Source: CAD feature listing. Evaluate the final solid. Frame: model axes, mm. A direction names the side the tool comes from. Give positions to 0.01 mm unless a question says otherwise; leave off trailing zeros. Order: outer loops, then holes, each group sorted by start corner. A loop starts at its lowest first (then second) coordinate and runs counter-clockwise, first axis right, second up. Notation, with made-up numbers: (-22.75, 62) -> (2.25, 62) arc R22 cw to (2.25, 84) -> close; hole circle Ø6 at (79, -27.5). An arc over 180 degrees is marked (long way). Use one line per item in the form item = value. Start each with the question number.
from build123d import *

# Parameters (mm, degrees)
SKETCH1_W           = 18.4
SKETCH1_H           = 15.9
BOSS_EXTRUDE1_DEPTH = 1.5
SKETCH2_W           = 2.5
SKETCH2_H           = 15.2
BOSS_EXTRUDE2_DEPTH = 2.6
BOSS_EXTRUDE3_START = -5.1
SKETCH3_W           = 0.64
SKETCH3_H           = 0.64
BOSS_EXTRUDE3_DEPTH = 11
SKETCH5_W           = 4.4
SKETCH5_H           = 5.1
SKETCH5_W_2         = 1.2
SKETCH5_H_2         = 2
BOSS_EXTRUDE4_DEPTH = 1.1
SKETCH6_W           = 1.2
SKETCH6_H           = 1.2
BOSS_EXTRUDE5_DEPTH = 1
SKETCH7_W           = 3.4
SKETCH7_H           = 1.8
BOSS_EXTRUDE6_DEPTH = 1.9
SKETCH8_W           = 1.2
SKETCH8_H           = 1.2
CUT_EXTRUDE1_DEPTH  = 0.05
SKETCH9_W           = 1.2
SKETCH9_H           = 1.05
CUT_EXTRUDE2_DEPTH  = 0.05
SKETCH10_W          = 1.2
SKETCH10_H          = 1.05
CUT_EXTRUDE3_DEPTH  = 0.05


with BuildPart() as part:
    # Sketch1 → Boss-Extrude1 (new body)
    with BuildSketch(Plane(origin=(0, 0, 0), x_dir=(1, 0, 0), z_dir=(0, 1, 0))):
        Rectangle(SKETCH1_W, SKETCH1_H)
    extrude(amount=-BOSS_EXTRUDE1_DEPTH)

    # Sketch2 → Boss-Extrude2 (add)
    with BuildSketch(Plane.XZ.offset(1.5)):
        with Locations((-7.6, 0)):
            Rectangle(SKETCH2_W, SKETCH2_H)
    boss_extrude2 = extrude(amount=BOSS_EXTRUDE2_DEPTH)

    # Sketch3 → Boss-Extrude3 (add)
    with BuildSketch(Plane(origin=(0, -4.1, 0), x_dir=(-1, 0, 0), z_dir=(0, -1, 0)).offset(BOSS_EXTRUDE3_START)):
        with Locations((7.6, -6.35)):
            Rectangle(SKETCH3_W, SKETCH3_H)
        with Locations((7.6, -3.81)):
            Rectangle(SKETCH3_W, SKETCH3_H)
        with Locations((7.6, -1.27)):
            Rectangle(SKETCH3_W, SKETCH3_H)
        with Locations((7.6, 1.27)):
            Rectangle(SKETCH3_W, SKETCH3_H)
        with Locations((7.6, 6.35)):
            Rectangle(SKETCH3_W, SKETCH3_H)
        with Locations((7.6, 3.81)):
            Rectangle(SKETCH3_W, SKETCH3_H)
    boss_extrude3 = extrude(amount=BOSS_EXTRUDE3_DEPTH)

    # Mirror1: Boss-Extrude2, Boss-Extrude3 across plane
    add(boss_extrude2.mirror(Plane(origin=(0, 0, 0), x_dir=(0, 0, 1), z_dir=(1, 0, 0))))
    add(boss_extrude3.mirror(Plane(origin=(0, 0, 0), x_dir=(0, 0, 1), z_dir=(1, 0, 0))))

    # Sketch5 → Boss-Extrude4 (add)
    with BuildSketch(Plane(origin=(0, 0, 0), x_dir=(1, 0, 0), z_dir=(0, 1, 0))):
        with Locations((-1.5, 0.5)):
            Rectangle(SKETCH5_W, SKETCH5_H)
        with Locations((4.5979, 0.1395)):
            Rectangle(SKETCH5_W_2, SKETCH5_H_2)
        with Locations((4.5979, 5.5766)):
            Rectangle(SKETCH5_W_2, SKETCH5_H_2)
    extrude(amount=BOSS_EXTRUDE4_DEPTH)

    # Sketch6 → Boss-Extrude5 (add)
    with BuildSketch(Plane(origin=(0, 0, 0), x_dir=(1, 0, 0), z_dir=(0, 1, 0))):
        with Locations((-0.3788, 6.0122)):
            Rectangle(SKETCH6_W, SKETCH6_H)
    extrude(amount=BOSS_EXTRUDE5_DEPTH)

    # Sketch7 → Boss-Extrude6 (add)
    with BuildSketch(Plane(origin=(0, 0, 0), x_dir=(1, 0, 0), z_dir=(0, 1, 0))):
        with Locations((-2.8238, -5.3484)):
            Rectangle(SKETCH7_W, SKETCH7_H)
    extrude(amount=BOSS_EXTRUDE6_DEPTH)

    # Sketch8 → Cut-Extrude1 (cut)
    with BuildSketch(Plane(origin=(0, 1.1, 0), x_dir=(1, 0, 0), z_dir=(0, 1, 0))):
        with Locations((4.5979, 5.5766)):
            Rectangle(SKETCH8_W, SKETCH8_H)
        with Locations((4.5979, 0.1395)):
            Rectangle(SKETCH8_W, SKETCH8_H)
    extrude(amount=-CUT_EXTRUDE1_DEPTH, mode=Mode.SUBTRACT)

    # Sketch9 → Cut-Extrude2 (cut)
    with BuildSketch(Plane.ZY.offset(-3.9979)):
        with Locations((-0.1395, 0.525)):
            Rectangle(SKETCH9_W, SKETCH9_H)
        with Locations((-5.5766, 0.525)):
            Rectangle(SKETCH9_W, SKETCH9_H)
    extrude(amount=-CUT_EXTRUDE2_DEPTH, mode=Mode.SUBTRACT)

    # Sketch10 → Cut-Extrude3 (cut)
    with BuildSketch(Plane(origin=(5.1979, 0, 0), x_dir=(0, 0, -1), z_dir=(1, 0, 0))):
        with Locations((0.1395, 0.525)):
            Rectangle(SKETCH10_W, SKETCH10_H)
        with Locations((5.5766, 0.525)):
            Rectangle(SKETCH10_W, SKETCH10_H)
    extrude(amount=-CUT_EXTRUDE3_DEPTH, mode=Mode.SUBTRACT)


solid = part.part
1) Cut plane B-B, the plane z = -2.25. Return the cut outline in (x, y), plus the area to 3 significant figures.
2) Reachability of faces 1 (the face through (4.6, 0.5, -4.577)), 2 (the face through (4.6, 0.5, -6.577)), 3 (the face through (0.7, 0.5, -0.5)), 4 (the face through (-2, 1.1, -1)), 5 (the face through (0, 1, -6)) from +Z, -Z, +X, -X, +Y, -Y: full face, straight path, thin tool, end or side. Return the list, or none.
3) Cut plane C-C, the plane x = -1.5. Return the cut outline in (y, z), plus the area to 3 significant figures.
4) Material intervals for probe 1 along X at (y, z) = (0.25, -6.5); probe 2 along X at (y, z) = (-1.75, 4); probe 3 along Y at (x, z) = (2, 7), sorted ascending.
5) Draft query along X for faces 6 (the face through (8.85, -3, 0)), 7 (the face through (6.35, -3, 0)), 8 (the face through (4.6, 1.05, -0.1)), 9 (the face through (-3.7, 0.5, -0.5)). Return one class per face: +X half, -X half, draft (parallel to the pull), parting line (faces both ways), or undercut.
6) Pin query (flat end, axial travel): pin 1 (1.5 mm diameter, centred on y = -2.5, z = 0.5, fed in from -X); pin 2 (4 mm diameter, centred on x = -1.5, z = 5.5, fed in from -Y); pin 3 (0.5 mm diameter, centred on y = 0.5, z = -6.5, fed in from +X). Return the tip coordinate at first contact, or that it passes through.
7) Cut plane A-A, the plane y = -3.75. Return the cut outline in (x, z).
8) Cut plane D-D, the plane x = 4.5. Return the cut outline in (y, z), plus the area to 3 significant figures.
Output values:
q1.outline = (-9.2, -1.5) -> (-8.85, -1.5) -> (-8.85, -4.1) -> (-6.35, -4.1) -> (-6.35, -1.5) -> (6.35, -1.5) -> (6.35, -4.1) -> (8.85, -4.1) -> (8.85, -1.5) -> (9.2, -1.5) -> (9.2, 0) -> (0.7, 0) -> (0.7, 1.1) -> (-3.7, 1.1) -> (-3.7, 0) -> (-9.2, 0) -> close
q1.area = 45.4 mm^2
q2.face_1 = +X, -X, +Y
q2.face_2 = -Z, +Y
q2.face_3 = +Z, -Z, +Y
q2.face_4 = -Z, +X, -X, +Y
q2.face_5 = -Z, -X, +Y
q3.outline = (-1.5, -7.95) -> (0, -7.95) -> (0, -3.05) -> (1.1, -3.05) -> (1.1, 2.05) -> (0, 2.05) -> (0, 4.45) -> (1.9, 4.45) -> (1.9, 6.25) -> (0, 6.25) -> (0, 7.95) -> (-1.5, 7.95) -> close
q3.area = 32.9 mm^2
q4.probe_1 = -7.92 to -7.28, -0.98 to 0.22, 4 to 5.2, 7.28 to 7.92
q4.probe_2 = -8.85 to -6.35, 6.35 to 8.85
q4.probe_3 = -1.5 to 0
q5.face_6 = +X half
q5.face_7 = undercut
q5.face_8 = draft
q5.face_9 = undercut
q6.pin_1 = -8.85
q6.pin_2 = -1.5
q6.pin_3 = 7.92
q7.outline = (-8.85, -7.6) -> (-6.35, -7.6) -> (-6.35, 7.6) -> (-8.85, 7.6) -> close; (6.35, -7.6) -> (8.85, -7.6) -> (8.85, 7.6) -> (6.35, 7.6) -> close
q8.outline = (-1.5, -7.95) -> (0, -7.95) -> (0, -6.58) -> (1.1, -6.58) -> (1.1, -6.18) -> (1.05, -6.18) -> (1.05, -4.98) -> (1.1, -4.98) -> (1.1, -4.58) -> (0, -4.58) -> (0, -1.14) -> (1.1, -1.14) -> (1.1, -0.74) -> (1.05, -0.74) -> (1.05, 0.46) -> (1.1, 0.46) -> (1.1, 0.86) -> (0, 0.86) -> (0, 7.95) -> (-1.5, 7.95) -> close
q8.area = 28.1 mm^2
